```python
from build123d import *

# Parameters (mm, degrees)
F0_W     = 127.4
F0_H     = 152.4
F0_W_2   = 125
F0_H_2   = 150
F1_DEPTH = 1.2
F2_DEPTH = 6.2
F3_W     = 108
F3_H     = 64.8
F4_DEPTH = 1.2
F3_R     = 1.5
F5_DEPTH = 4.1
F6_R     = 2
F3_W_2   = 124
F3_H_2   = 35
F7_DEPTH = 1.2
F8_DEPTH = 5


with BuildPart() as f1:
    # F0 (on Front) → F1 (new body)
    with BuildSketch(Plane.XZ):
        with Locations((62.5, -75)):
            Rectangle(F0_W, F0_H)
        with Locations((62.5, -75)):
            Rectangle(F0_W_2, F0_H_2, mode=Mode.SUBTRACT)
        with Locations((62.5, -75)):
            Rectangle(F0_W_2, F0_H_2)
    extrude(amount=F1_DEPTH)

    # F0 (on Front) → F2 (join)
    with BuildSketch(Plane.XZ):
        with Locations((62.5, -75)):
            Rectangle(F0_W, F0_H)
        with Locations((62.5, -75)):
            Rectangle(F0_W_2, F0_H_2, mode=Mode.SUBTRACT)
    extrude(amount=F2_DEPTH)

    # F3 (on face) → F4 (cut)
    with BuildSketch(Plane.XZ.offset(1.2)):
        with Locations((62.5, -43.917)):
            Rectangle(F3_W, F3_H)
    extrude(amount=-F4_DEPTH, mode=Mode.SUBTRACT)

    # F3 (on face) → F5 (join)
    with BuildSketch(Plane.XZ.offset(1.2)):
        with BuildLine():
            Line((2.15, -4.27), (2.15, -8.147))
            Line((2.15, -8.147), (9.897, -8.147))
            Line((9.897, -8.147), (9.897, -4.27))
            ThreePointArc((9.897, -4.27), (8.763503, -1.533497), (6.027, -0.4))
            Line((6.027, -0.4), (6.02, -0.4))
            ThreePointArc((6.02, -0.4), (3.283497, -1.533497), (2.15, -4.27))
        make_face()
        with Locations((6.0235, -4.2735)):
            Circle(F3_R, mode=Mode.SUBTRACT)
        with BuildLine():
            Line((115.103, -4.27), (115.103, -8.147))
            Line((115.103, -8.147), (122.85, -8.147))
            Line((122.85, -8.147), (122.85, -4.27))
            ThreePointArc((122.85, -4.27), (121.716503, -1.533497), (118.98, -0.4))
            Line((118.98, -0.4), (118.973, -0.4))
            ThreePointArc((118.973, -0.4), (116.236497, -1.533497), (115.103, -4.27))
        make_face()
        with Locations((118.9765, -4.2735)):
            Circle(F3_R, mode=Mode.SUBTRACT)
        with BuildLine():
            Line((122.85, -83.947), (115.103, -83.947))
            Line((115.103, -83.947), (115.103, -87.824))
            ThreePointArc((115.103, -87.824), (116.236497, -90.560503), (118.973, -91.694))
            Line((118.973, -91.694), (118.98, -91.694))
            ThreePointArc((118.98, -91.694), (121.716503, -90.560503), (122.85, -87.824))
            Line((122.85, -87.824), (122.85, -83.947))
        make_face()
        with Locations((118.9765, -87.8205)):
            Circle(F3_R, mode=Mode.SUBTRACT)
        with BuildLine():
            Line((9.897, -83.947), (2.15, -83.947))
            Line((2.15, -83.947), (2.15, -87.824))
            ThreePointArc((2.15, -87.824), (3.283497, -90.560503), (6.02, -91.694))
            Line((6.02, -91.694), (6.027, -91.694))
            ThreePointArc((6.027, -91.694), (8.763503, -90.560503), (9.897, -87.824))
            Line((9.897, -87.824), (9.897, -83.947))
        make_face()
        with Locations((6.0235, -87.8205)):
            Circle(F3_R, mode=Mode.SUBTRACT)
    extrude(amount=F5_DEPTH)

    # F6
    f6_edges = [f1.edges().sort_by_distance(p)[0] for p in [
        (126.2, -3.1, -151.2),
        (126.2, -3.1, 1.2),
        (-1.2, -3.1, 1.2),
        (-1.2, -3.1, -151.2),
    ]]
    fillet(f6_edges, radius=F6_R)

    # F3 (on face) → F7 (cut)
    with BuildSketch(Plane.XZ.offset(1.2)):
        with Locations((62.5, -116.33127)):
            Rectangle(F3_W_2, F3_H_2)
    extrude(amount=-F7_DEPTH, mode=Mode.SUBTRACT)

    # F3 (on face) → F8 (join)
    with BuildSketch(Plane.XZ.offset(1.2)):
        with BuildLine():
            Line((125, -150), (125, -144))
            Line((125, -144), (122, -144))
            ThreePointArc((122, -144), (119.87868, -144.87868), (119, -147))
            Line((119, -147), (119, -150))
            Line((119, -150), (125, -150))
        make_face()
        with Locations((122, -147)):
            Circle(F3_R, mode=Mode.SUBTRACT)
        with BuildLine():
            Line((0, -144), (0, -150))
            Line((0, -150), (6, -150))
            Line((6, -150), (6, -147))
            ThreePointArc((6, -147), (5.12132, -144.87868), (3, -144))
            Line((3, -144), (0, -144))
        make_face()
        with Locations((3, -147)):
            Circle(F3_R, mode=Mode.SUBTRACT)
    extrude(amount=F8_DEPTH)


solid = f1.part
```
Work out the finished part from the listing and answer in its coordinate system (mm). Coordinates: 2 decimals unless noted, no trailing zeros. Loops run counter-clockwise (first coordinate to the right, second up) from the corner with the lowest first, then second, coordinate; pieces in that order, holes last. Notation, with made-up numbers: (54, -25) - (81, -25) arc R17 cw to (81, -3) - close; hole circle Ø5 at (50.5, -24). An arc over 180 degrees is marked (long way). Use a Markdown table: item, result.
Item 1: Find section A-A, the plane z = -116. Determine the outline of the cut face in (x, y).
Evaluation:
| item | result |
|---|---|
| outline | (-1.2, -6.2) - (0, -6.2) - (0, -1.2) - (0.5, -1.2) - (0.5, 0) - (-1.2, 0) - close; (124.5, -1.2) - (125, -1.2) - (125, -6.2) - (126.2, -6.2) - (126.2, 0) - (124.5, 0) - close |
Item 2: Find section B-B, the plane x = 86.5. Determine the outline of the cut face in (y, z).
Evaluation:
| item | result |
|---|---|
| outline | (-6.2, -151.2) - (0, -151.2) - (0, -133.83) - (-1.2, -133.83) - (-1.2, -150) - (-6.2, -150) - close; (-6.2, 0) - (-1.2, 0) - (-1.2, -11.52) - (0, -11.52) - (0, 1.2) - (-6.2, 1.2) - close; (-1.2, -98.83) - (0, -98.83) - (0, -76.32) - (-1.2, -76.32) - close |
Item 3: Given pin 1 Ø0.9 at (x, z) = (119, -4) entering from -Y; pin 2 Ø2.5 at (x, z) = (7, -5) entering from -Y, each flat-ended and moving along its own axis, determine where each tip first touches the part or whether it passes through.
Evaluation:
| item | result |
|---|---|
| pin 1 | stops at y = -1.2 |
| pin 2 | stops at y = -5.3 |
Item 4: Find section C-C, the plane y = -3.25. State how many separate pieces and enclosed holes the cut face has, and give its area (3 significant figures).
Evaluation:
| item | result |
|---|---|
| separate pieces | 5 |
| enclosed holes | 7 |
| area | 902 mm2 |
Item 5: Find section D-D, the plane z = -67. Determine the outline of the cut face in (x, y), and give its area (3 significant figures).
Evaluation:
| item | result |
|---|---|
| outline | (-1.2, -6.2) - (0, -6.2) - (0, -1.2) - (8.5, -1.2) - (8.5, 0) - (-1.2, 0) - close; (116.5, -1.2) - (125, -1.2) - (125, -6.2) - (126.2, -6.2) - (126.2, 0) - (116.5, 0) - close |
| area | 35.3 mm2 |
Item 6: The mould has two halves that part along Z. Classify faces 1 (the flat face through (119, -1.2, -4)), 2 (the flat face through (62, -3, -151.2)), 3 (the flat face through (62, 0, -91)), 4 (the flat face through (6, -5.3, -86)): +Z half, -Z half, draft (parallel to the pull), parting line (faces both ways), or undercut.
Evaluation:
| item | result |
|---|---|
| face 1 | undercut |
| face 2 | -Z half |
| face 3 | draft |
| face 4 | undercut |
Item 7: Consider probe 1 along Z at (x, y) = (32, -0.75); probe 2 along X at (y, z) = (-3.5, -147); probe 3 along X at (y, z) = (-5.5, -31.5). Determine where each line is inside the solid, lowest interval first. Write a range as from..to.
Evaluation:
| item | result |
|---|---|
| probe 1 | z = -151.2..-133.83, -98.83..-76.32, -11.52..1.2 |
| probe 2 | x = -1.2..1.5, 4.5..6, 119..120.5, 123.5..126.2 |
| probe 3 | x = -1.2..0, 125..126.2 |
